```python
from build123d import *
from build123d.topology import SkipClean

# Parameters (mm, degrees)
REVOLU_O1_ANGLE            = 90
ESBO_O3_R                  = 2.5
CORTE_EXTRUS_O1_DEPTH      = 79.698792875
RESSALTO_EXTRUS_O1_START   = 13
ESBO_O7_R                  = 2.5
RESSALTO_EXTRUS_O1_DEPTH   = 13
CORTE_EXTRUS_O3_DEPTH      = 79.698792875
CORTE_EXTRUS_O3_DEPTH_BACK = 6.5
ESBO_O4_R                  = 3.5
ESBO_O6_R                  = 1.75
CORTE_EXTRUS_O4_DEPTH      = 71.924255371
CORTE_EXTRUS_O5_START      = -6.5
ESBO_O8_R                  = 3.1
CORTE_EXTRUS_O5_DEPTH      = 13
CHANFRO1_SIZE              = 2
CORTE_EXTRUS_O6_DEPTH      = 82.701335058
CORTE_EXTRUS_O7_DEPTH      = 81.405896153


with BuildPart() as part:
    # Esboço2 → Revolução1 (revolve)
    with BuildSketch(Plane.XY):
        with BuildLine():
            Line((-23.5, 42.5), (-23.5, 68.5))
            ThreePointArc((-23.5, 68.5), (-36.5, 55.5), (-23.5, 42.5))
        make_face()
    revolve(axis=Axis((-23.5, 42.5, 0), (0, 1, 0)), revolution_arc=REVOLU_O1_ANGLE)

    # Esboço3 → Corte-extrusão1 (cut, through all)
    with BuildSketch(Plane.XY):
        with Locations(Location((-29.2, 62, 0), (0, 0, 142.736397609))):
            Circle(ESBO_O3_R)
        with Locations(Location((-29.2, 49, 0), (0, 0, 233.94500715))):
            Circle(ESBO_O3_R)
    extrude(amount=CORTE_EXTRUS_O1_DEPTH, mode=Mode.SUBTRACT)

    # Esboço7 → Ressalto-extrusão1 (add)
    with SkipClean():  # the faces are left unmerged after this step: merging them gives an invalid solid
        with BuildSketch(Plane(origin=(0, 0, 0), x_dir=(-1, 0, 0), z_dir=(0, 0, -1)).offset(RESSALTO_EXTRUS_O1_START)):
            with BuildLine():
                Line((23.5, 68.5), (23.5, 42.5))
                ThreePointArc((23.5, 42.5), (36.5, 55.5), (23.5, 68.5))
            make_face()
            with Locations((29.2, 62)):
                Circle(ESBO_O7_R, mode=Mode.SUBTRACT)
            with Locations((29.2, 49)):
                Circle(ESBO_O7_R, mode=Mode.SUBTRACT)
        extrude(amount=-RESSALTO_EXTRUS_O1_DEPTH)

    # Esboço4 → Corte-extrusão3 (cut, two sides: drawn at the far end of the back side and taken through both)
    with BuildSketch(Plane.XY.offset(-CORTE_EXTRUS_O3_DEPTH_BACK)):
        with Locations((-29.2, 62)):
            Circle(ESBO_O4_R)
        with Locations((-29.2, 49)):
            Circle(ESBO_O4_R)
    extrude(amount=CORTE_EXTRUS_O3_DEPTH + CORTE_EXTRUS_O3_DEPTH_BACK, mode=Mode.SUBTRACT)

    # Esboço6 → Corte-extrusão4 (cut, through all)
    with BuildSketch(Plane(origin=(-23.5, 0, 0), x_dir=(0, 0, -1), z_dir=(1, 0, 0))):
        with Locations((-0.5, 55.5)):
            Circle(ESBO_O6_R)
    extrude(amount=-CORTE_EXTRUS_O4_DEPTH, mode=Mode.SUBTRACT)

    # Esboço8 → Corte-extrusão5 (cut)
    with BuildSketch(Plane(origin=(-23.5, 0, 0), x_dir=(0, 0, -1), z_dir=(1, 0, 0)).offset(CORTE_EXTRUS_O5_START)):
        with Locations(Location((-0.5, 55.5, 0), (0, 0, 279.281799091))):
            Circle(ESBO_O8_R)
    extrude(amount=-CORTE_EXTRUS_O5_DEPTH, mode=Mode.SUBTRACT)

    # Chanfro1
    # the kernel refuses this chamfer: 2 mm, written as the material it takes off along each edge
    with BuildSketch(Plane(origin=(-23.5, 42.5, -18.143365976), x_dir=(-0.9974093352150653, 0.07193481789677074, 0), z_dir=(0, 0, 1))) as chanfro1_piece_1:
        with BuildLine():
            Line((1.870305265, 0), (CHANFRO1_SIZE * 0.0719348178968, -CHANFRO1_SIZE * 0.997409335215))
            Line((CHANFRO1_SIZE * 0.0719348178968, -CHANFRO1_SIZE * 0.997409335215), (0, 0))
            ThreePointArc((0, 0), (0.961335866, 0.033652274), (1.870305265, 0))
        make_face()
    extrude(amount=18.143365976, mode=Mode.SUBTRACT)
    with BuildSketch(Plane(origin=(-23.5, 68.5, -18.143365976), x_dir=(-0.9974093352150653, -0.07193481789677116, 0), z_dir=(0, 0, 1))) as chanfro1_piece_2:
        with BuildLine():
            Line((1.870305265, 0), (CHANFRO1_SIZE * 0.0719348178968, CHANFRO1_SIZE * 0.997409335215))
            Line((CHANFRO1_SIZE * 0.0719348178968, CHANFRO1_SIZE * 0.997409335215), (0, 0))
            ThreePointArc((0, 0), (0.961335866, -0.033652274), (1.870305265, 0))
        make_face()
    extrude(amount=18.143365976, mode=Mode.SUBTRACT)
    with BuildSketch(Plane(origin=(-23.5, 55.5, 0), x_dir=(0, 1, 0), z_dir=(0, 0, -1))) as chanfro1_piece_3:
        with BuildLine():
            Line((12.865459931, -1.865459931), (13 - CHANFRO1_SIZE, 0))
            Line((13 - CHANFRO1_SIZE, 0), (13, 0))
            ThreePointArc((13, 0), (12.964411572, -0.961266138), (12.865459931, -1.865459931))
        make_face()
    revolve(axis=Axis((-23.5, 55.5, 0), (1, 0, 0)), revolution_arc=180, mode=Mode.SUBTRACT)

    # Esboço9 → Corte-extrusão6 (cut, through all)
    with BuildSketch(Plane(origin=(0, 0, -13), x_dir=(-1, 0, 0), z_dir=(0, 0, -1))):
        with BuildLine():
            Line((33.5, 47.193376137), (33.5, 63.806623863))
            ThreePointArc((33.5, 63.806623863), (36.5, 55.5), (33.5, 47.193376137))
        make_face()
    extrude(amount=-CORTE_EXTRUS_O6_DEPTH, mode=Mode.SUBTRACT)

    # Esboço10 → Corte-extrusão7 (cut, through all)
    with BuildSketch(Plane(origin=(0, 0, -13), x_dir=(-1, 0, 0), z_dir=(0, 0, -1))):
        Polygon((25, 68), (25, 43), (23.5, 44.5), (23.5, 66.5), align=None)
    extrude(amount=-CORTE_EXTRUS_O7_DEPTH, mode=Mode.SUBTRACT)


solid = part.part
```
For this review, take the finished solid that the model builds, in its own axes (mm). A direction names the side the tool comes from. Coordinates: 2 decimals unless noted, no trailing zeros. Order: outer loops, then holes, each group sorted by start corner. A loop starts at its lowest first (then second) coordinate and runs counter-clockwise, first axis right, second up. Notation, with made-up numbers: (33.25, 27) - (54.25, 27) arc R22 cw to (54.25, 60) - close; hole circle Ø5 at (85.5, 1). An arc over 180 degrees is marked (long way). Answer as a JSON object with one key per item and string values. Group by question number.
1. We need section A-A on z = -11.5. State the section outline as (x, y) points, then the cut area to 3 significant figures.
2. We need section B-B on y = 55.5. State the section outline as (x, z) points.
3. For faces 5 (the flat face through (-30, 54, 2)), 6 (the cylindrical face through (-29.91, 66.81, -6.59)), 7 (the cylindrical face through (-27.585, 58.895, 0.541)), list the 3-axis set-ups (+Z, -Z, +X, -X, +Y, -Y) from which the entire face can be reached by the end or side of a thin tool; tool diameter is ignored.
4. We need section D-D on x = -27. State the section outline as (y, z) points.
5. Clearance check with flat-ended pins moving along their axes: P1, Ø1.9, axis at y = 55, z = 1.5, coming from the -X side; P2, Ø5, axis at x = -27, z = 9.5, coming from the +Y side; P3, Ø1.5, axis at x = -29.5, z = -5.5, coming from the +Y side. State where each tip first meets the part, or that it passes through.
6. We need section C-C on x = -29.2. State the section outline as (y, z) points.
7. For probe 1 along X at (y, z) = (62, 1); probe 2 along Y at (x, z) = (-31.7, 0.5); probe 3 along Y at (x, z) = (-29, -0.5), list the stretches that pass through material, from the lowest coordinate up.
8. The part is to be moulded in two halves that separate along Z. For faces 1 (the cylindrical face through (-31.725, 52.482, 1.21)), 2 (the cylindrical face through (-26.7, 49.1, -9.8)), 3 (the flat face through (-29, 56, -13)), 4 (the conical face through (-25.14, 55.778, 12.637)), say which applies: pulls with the +Z half, pulls with the -Z half, needs draft (parallel to the pull), parting line crosses it, or undercut.
Final values:
{
 "1": {"outline": "(-33.5, 47.19) arc R13 ccw to (-25.37, 42.63) - (-25, 43) - (-25, 68) - (-25.37, 68.37) arc R13 ccw to (-33.5, 63.81) - close; hole circle Ø5 at (-29.2, 49); hole circle Ø5 at (-29.2, 62)", "area": "153 mm²"},
 "2": {"outline": "(-33.5, -13) - (-25, -13) - (-25, -1.25) - (-30, -1.25) - (-30, -2.6) - (-33.5, -2.6) - close; (-33.5, 3.6) - (-30, 3.6) - (-30, 2.25) - (-25, 2.25) - (-25, 12.5) - (-25.37, 12.87) arc R13 ccw to (-33.5, 8.31) - close"},
 "3": {"face 5": "-X", "face 6": "+Z, -Z, -X, +Y", "face 7": "+Z"},
 "4": {"outline": "(42.98, -13) - (47.81, -13) - (47.81, -6.5) - (46.28, -6.5) - (46.28, 8.47) arc R12.52 ccw to (42.98, 0) - close; (50.19, -13) - (60.81, -13) - (60.81, -6.5) - (59.28, -6.5) - (59.28, 11.94) arc R12.52 ccw to (51.72, 11.94) - (51.72, -6.5) - (50.19, -6.5) - close; (63.19, -13) - (68.02, -13) - (68.02, 0) arc R12.52 ccw to (64.72, 8.47) - (64.72, -6.5) - (63.19, -6.5) - close; hole circle Ø3.5 at (55.5, 0.5)"},
 "5": {"P1": "x = -30", "P2": "y = 66.03", "P3": "y = 67.39"},
 "6": {"outline": "(43.82, -13) - (46.5, -13) - (46.5, -6.5) - (45.5, -6.5) - (45.5, 6.04) arc R11.68 ccw to (43.82, 0) - close; (51.5, -13) - (59.5, -13) - (59.5, -6.5) - (58.5, -6.5) - (58.5, 11.29) arc R11.68 ccw to (52.5, 11.29) - (52.5, -6.5) - (51.5, -6.5) - close; (64.5, -13) - (67.18, -13) - (67.18, 0) arc R11.68 ccw to (65.5, 6.04) - (65.5, -6.5) - (64.5, -6.5) - close; hole circle Ø3.5 at (55.5, 0.5)"},
 "7": {"probe 1": "-33.5 to -32.7, -25.7 to -25", "probe 2": "45.42 to 46.55, 51.45 to 52.4, 58.6 to 59.55, 64.45 to 65.58", "probe 3": "43.72 to 45.51, 52.49 to 54.06, 56.94 to 58.51, 65.49 to 67.28"},
 "8": {"face 1": "undercut", "face 2": "needs draft", "face 3": "pulls with the -Z half", "face 4": "pulls with the +Z half"}
}
